```python
from build123d import *

# Parameters (mm, degrees)
F1_DEPTH    = 17.5
F2_R        = 2.5
F3_DEPTH    = 335
F4_T1_DEPTH = 56.5
F4_T3_DEPTH = 56.5


# Not quite as in the source:
# - a fillet or chamfer that OpenCascade refuses, or shapes differently, is made with other operations: its cross-section is extruded or revolved along the edge and cut away or added


with BuildPart() as f1:
    # F0 (on Front) → F1 (new body)
    with BuildSketch(Plane.XZ):
        Polygon((-146, -137.7746703387), (0, -137.7746703387), (146, -137.7746703387), (146, -199), (157.5, -199), (157.5, 0), (157.5, 199), (146, 199), (146, 0), (146, -126.2746703387), (8.7075978518, -126.2746703387), (0, -126.2746703387), (-6.4604924992, -126.2746703387), (-146, -126.2746703387), (-146, 0), (-146, 199), (-157.5, 199), (-157.5, 0), (-157.5, -199), (-146, -199), align=None)
    extrude(amount=F1_DEPTH)

    # F2 (on face) → F3 (cut)
    with BuildSketch(Plane(origin=(-157.5, 0, 0), x_dir=(0, -1, 0), z_dir=(-1, 0, 0))):
        with Locations((8.75, -190.25)):
            Circle(F2_R)
    extrude(amount=-F3_DEPTH, mode=Mode.SUBTRACT)

    # F4: fillet of radius 9 on 4 edges, made by hand

    # F4_s2 → F4_t1 (cut)
    with BuildSketch(Plane.YZ.offset(-180)):
        with BuildLine():
            ThreePointArc((0, -190), (-2.6360389693, -196.3639610307), (-9, -199))
            Line((-9, -199), (0, -199))
            Line((0, -199), (0, -190))
        make_face()
        with BuildLine():
            ThreePointArc((-17.5, -190), (-14.8639610307, -196.3639610307), (-8.5, -199))
            Line((-8.5, -199), (-17.5, -199))
            Line((-17.5, -199), (-17.5, -190))
        make_face()
    extrude(amount=F4_T1_DEPTH, mode=Mode.SUBTRACT)

    # F4_s4 → F4_t3 (cut)
    with BuildSketch(Plane.YZ.offset(123.5)):
        with BuildLine():
            ThreePointArc((0, -190), (-2.6360389693, -196.3639610307), (-9, -199))
            Line((-9, -199), (0, -199))
            Line((0, -199), (0, -190))
        make_face()
        with BuildLine():
            ThreePointArc((-17.5, -190), (-14.8639610307, -196.3639610307), (-8.5, -199))
            Line((-8.5, -199), (-17.5, -199))
            Line((-17.5, -199), (-17.5, -190))
        make_face()
    extrude(amount=F4_T3_DEPTH, mode=Mode.SUBTRACT)


solid = f1.part
```
The listing builds one solid part. Answer for the finished solid, in the listing's coordinates (mm). A direction names the side the tool comes from. Round coordinates to 2 decimals unless told otherwise and drop trailing zeros. Loops run counter-clockwise (first coordinate to the right, second up) from the corner with the lowest first, then second, coordinate; pieces in that order, holes last. Notation, with made-up numbers: (50.5, 57) - (61.5, 57) arc R30 ccw to (61.5, 80) - close; hole circle Ø1 at (18.25, 5). An arc over 180 degrees is marked (long way). Return JSON: item names as keys, results as strings. Group by question number.
1. The part is cut by section C-C on x = 81.5. Determine the outline of the cut face in (y, z).
2. Which of the six approach directions +Z, -Z, +X, -X, +Y, -Y give full straight-line access (tool end or side, diameter ignored) to faces 5 (the flat face through (151, -17.5, 5)), 6 (the flat face through (2, -9, -126.275)), 7 (the flat face through (-2, -9, -137.775))?
3. The part is cut by section A-A on z = -19.5. Determine the outline of the cut face in (x, y).
4. The part is cut by section B-B on y = -3.25. Determine the outline of the cut face in (x, z).
5. Each of these flat-tipped pins is pushed along its axis until it touches: P1, Ø5, axis at x = 73.5, y = -11, coming from the +Z side; P2, Ø4, axis at y = -8.75, z = -190.25, coming from the -X side (3 decimals); P3, Ø9, axis at x = -3, y = -9, coming from the -Z side. Where does it stop, or does it pass through?
6. Consider probe 1 along Z at (x, y) = (-151.5, -8.75); probe 2 along X at (y, z) = (-3.5, -83.5); probe 3 along Y at (x, z) = (150.5, -190.25). Determine where each line is inside the solid, lowest interval first.
7. The mould has two halves that part along X. Classify faces 1 (the flat face through (-146, -9, 34)), 2 (the flat face through (157.5, -9, -3)), 3 (the flat face through (-157.5, -9, 3)), 4 (the cylindrical face through (-151.83, -15.019, -196.205)): pulls with the +X half, pulls with the -X half, needs draft (parallel to the pull), parting line crosses it, or undercut.
Resolved:
{
 "1": {"outline": "(-17.5, -137.77) - (0, -137.77) - (0, -126.27) - (-17.5, -126.27) - close"},
 "2": {"face 5": "+Z, -Z, +X, -X, -Y", "face 6": "+Z, +Y, -Y", "face 7": "-Z, +Y, -Y"},
 "3": {"outline": "(-157.5, -17.5) - (-146, -17.5) - (-146, 0) - (-157.5, 0) - close; (146, -17.5) - (157.5, -17.5) - (157.5, 0) - (146, 0) - close"},
 "4": {"outline": "(-157.5, -196.92) - (-146, -196.92) - (-146, -137.77) - (146, -137.77) - (146, -196.92) - (157.5, -196.92) - (157.5, 199) - (146, 199) - (146, -126.27) - (-146, -126.27) - (-146, 199) - (-157.5, 199) - close"},
 "5": {"P1": "stops at z = -126.27", "P2": "passes through", "P3": "stops at z = -137.77"},
 "6": {"probe 1": "z = -199 to -192.75, -187.75 to 199", "probe 2": "x = -157.5 to -146, 146 to 157.5", "probe 3": "y = -17.5 to -11.25, -6.25 to 0"},
 "7": {"face 1": "undercut", "face 2": "pulls with the +X half", "face 3": "pulls with the -X half", "face 4": "needs draft"}
}
